Here's how the part is built. I have some questions about the finished solid (model axes, mm). A direction names the side the tool comes from. Give positions to 0.01 mm unless a question says otherwise; leave off trailing zeros. Loops run counter-clockwise (first coordinate to the right, second up) from the corner with the lowest first, then second, coordinate; pieces in that order, holes last. Notation, with made-up numbers: (72.5, 85.25) -> (82.5, 85.25) arc R33 ccw to (82.5, 114.25) -> close; hole circle Ø1 at (1, -7.5). An arc over 180 degrees is marked (long way). Answer in a Markdown table with one row per item. Add a question column.
Item 1: If I drill on line 1 (X direction, y = 42.75, z = -49.5); line 2 (Z direction, x = 4, y = 48.5); line 3 (Z direction, x = -14.5, y = 46.25), over which ranges is the centre line in solid material (lowest first)?
Item 2: If we section it at A-A (z = -11.5): Write out the boundary of the cut face in (x, y), then the cut area to 3 significant figures.
Item 3: If we section it at C-C (x = -6.5): Write out the boundary of the cut face in (y, z), then the cut area to 3 significant figures.
Item 4: We'd pull the mould along X, two halves only. Please class faces 4 (the face through (9, 43, 0)), 5 (the face through (13.468, 43, -36)), 6 (the face through (-24.532, 43, -35)): released by +X, released by -X, zero draft, split by the parting line, or undercut.
Item 5: For P1, Ø7.5, axis at x = -13.5, y = 40.5, coming from the +Z side, with a flat end and sliding along its axis, tell me the tip position at first contact or that it passes through.
Item 6: Which directions (+Z, -Z, +X, -X, +Y, -Y) give clear straight access to the entire face, cutting with the end or side of a thin tool? Please do faces 1 (the face through (-29.532, 43, -37)), 2 (the face through (3.468, 43, -1)), 3 (the face through (-22, 43, -3)).
Item 7: If we section it at B-B (y = 39): Write out the boundary of the cut face in (x, z).
Solid Edge part; units mm, degrees
sketch "Sketch1" plane through (0, 0, 0) normal (0, 0, 1) x (1, 0, 0)
  line L0 (-19.5323, 35.3812) -> (-19.5323, 50.3812)
  line L1 (-19.5323, 50.3812) -> (-24.5323, 50.3812)
  line L2 (-24.5323, 50.3812) -> (-24.5323, 35.3812)
  line L3 (-24.5323, 35.3812) -> (-19.5323, 35.3812)
  line L4 (8.4677, 50.3812) -> (8.4677, 35.3812)
  line L5 (8.4677, 35.3812) -> (3.4677, 35.3812)
  line L6 (3.4677, 35.3812) -> (3.4677, 50.3812)
  line L7 (3.4677, 50.3812) -> (8.4677, 50.3812)
extrude "Protrusion1" add sketch "Sketch1" against normal blind 3
sketch "Sketch2" plane through (0, 0, 0) normal (0, 0, 1) x (1, 0, 0)
  line L0 (13.4677, 35.3812) -> (13.4677, 50.3812)
  line L1 (13.4677, 50.3812) -> (8.4677, 50.3812)
  line L2 (8.4677, 50.3812) -> (8.4677, 35.3812)
  line L3 (8.4677, 35.3812) -> (13.4677, 35.3812)
  line L4 (-29.5323, 35.3812) -> (-24.5323, 35.3812)
  line L5 (-24.5323, 35.3812) -> (-24.5323, 50.3812)
  line L6 (-24.5323, 50.3812) -> (-29.5323, 50.3812)
  line L7 (-29.5323, 50.3812) -> (-29.5323, 35.3812)
extrude "Protrusion2" add sketch "Sketch2" against normal blind 68.5
sketch "Sketch3" plane through (13.4677, 42.8812, -34.25) normal (1, 0, 0) x (0, -1, 0)
  line L0 (7.5, 34.25) -> (7.5, 39.25)
  line L1 (7.5, 39.25) -> (-7.5, 39.25)
  line L2 (-7.5, 39.25) -> (-7.5, 34.25)
  line L3 (-7.5, 34.25) -> (7.5, 34.25)
extrude "Protrusion3" add sketch "Sketch3" against normal blind 43
Recorded:
| question | item | result |
|---|---|---|
| 1 | line 1 | x = -29.53 to -24.53, 8.47 to 13.47 |
| 1 | line 2 | z = -73.5 to -68.5, -3 to 0 |
| 1 | line 3 | z = -73.5 to -68.5 |
| 2 | outline | (-29.53, 35.38) -> (-24.53, 35.38) -> (-24.53, 50.38) -> (-29.53, 50.38) -> close; (8.47, 35.38) -> (13.47, 35.38) -> (13.47, 50.38) -> (8.47, 50.38) -> close |
| 2 | area | 150 mm^2 |
| 3 | outline | (35.38, -73.5) -> (50.38, -73.5) -> (50.38, -68.5) -> (35.38, -68.5) -> close |
| 3 | area | 75.0 mm^2 |
| 4 | face 4 | zero draft |
| 4 | face 5 | released by +X |
| 4 | face 6 | undercut |
| 5 | P1 | stops at z = -68.5 |
| 6 | face 1 | +Z, -Z, -X, +Y, -Y |
| 6 | face 2 | +Z, +Y, -Y |
| 6 | face 3 | +Y, -Y |
| 7 | outline | (-29.53, -73.5) -> (13.47, -73.5) -> (13.47, 0) -> (3.47, 0) -> (3.47, -3) -> (8.47, -3) -> (8.47, -68.5) -> (-24.53, -68.5) -> (-24.53, -3) -> (-19.53, -3) -> (-19.53, 0) -> (-29.53, 0) -> close |
